Geometry check sheet. Reference: the model listing, model coordinates, mm. Round coordinates to 2 decimals unless told otherwise and drop trailing zeros. Loops run counter-clockwise (first coordinate to the right, second up) from the corner with the lowest first, then second, coordinate; pieces in that order, holes last. Notation, with made-up numbers: (75.5, 65.25) -> (85.5, 65.25) arc R25 cw to (85.5, 82.25) -> close; hole circle Ø11 at (71, 25). An arc over 180 degrees is marked (long way). Use one line per item in the form item = value.
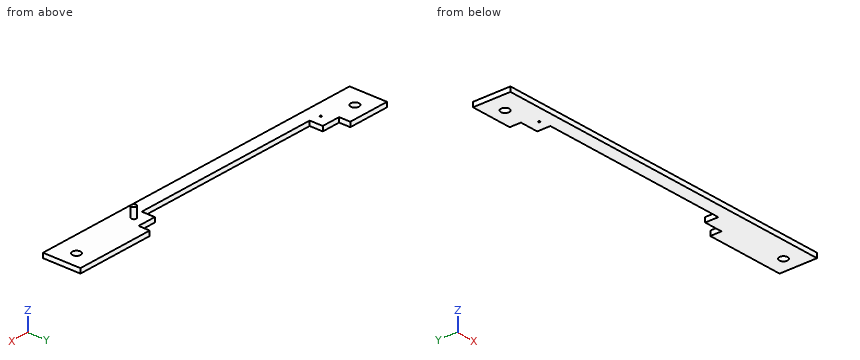
from build123d import *

# Parameters (mm, degrees)
BOX_W             = 188
BOX_H             = 20
BOX_DEPTH         = 2.5
CYLINDER_R        = 2.25
CYLINDER_DEPTH    = 2.5
CYLINDER001_R     = 2.25
CYLINDER001_DEPTH = 2.5
BOX001_W          = 123
BOX001_H          = 6
BOX001_DEPTH      = 2.5
BOX002_W          = 103
BOX002_H          = 7
BOX002_DEPTH      = 2.5
CYLINDER003_R     = 1.3
CYLINDER003_DEPTH = 6
CYLINDER004_R     = 0.5
CYLINDER004_DEPTH = 2.5


with BuildPart() as part:
    # Box → Box (join)
    with BuildSketch(Plane.XY):
        with Locations((94, 10)):
            Rectangle(BOX_W, BOX_H)
    extrude(amount=BOX_DEPTH)

    # Cylinder → Cylinder (cut)
    with BuildSketch(Plane(origin=(10.5, 12, 0), x_dir=(1, 0, 0), z_dir=(0, 0, 1))):
        Circle(CYLINDER_R)
    extrude(amount=CYLINDER_DEPTH, mode=Mode.SUBTRACT)

    # Cylinder001 → Cylinder001 (cut)
    with BuildSketch(Plane(origin=(179.5, 10.5, 0), x_dir=(1, 0, 0), z_dir=(0, 0, 1))):
        Circle(CYLINDER001_R)
    extrude(amount=CYLINDER001_DEPTH, mode=Mode.SUBTRACT)

    # Box001 → Box001 (cut)
    with BuildSketch(Plane(origin=(22.5, 14, 0), x_dir=(1, 0, 0), z_dir=(0, 0, 1))):
        with Locations((61.5, 3)):
            Rectangle(BOX001_W, BOX001_H)
    extrude(amount=BOX001_DEPTH, mode=Mode.SUBTRACT)

    # Box002 → Box002 (cut)
    with BuildSketch(Plane(origin=(32.5, 7, 0), x_dir=(1, 0, 0), z_dir=(0, 0, 1))):
        with Locations((51.5, 3.5)):
            Rectangle(BOX002_W, BOX002_H)
    extrude(amount=BOX002_DEPTH, mode=Mode.SUBTRACT)

    # Cylinder003 → Cylinder003 (join)
    with BuildSketch(Plane(origin=(141.5, 8, 2), x_dir=(1, 0, 0), z_dir=(0, 0, 1))):
        Circle(CYLINDER003_R)
    extrude(amount=CYLINDER003_DEPTH)

    # Cylinder004 → Cylinder004 (cut)
    with BuildSketch(Plane(origin=(26.75, 8, 0), x_dir=(1, 0, 0), z_dir=(0, 0, 1))):
        Circle(CYLINDER004_R)
    extrude(amount=CYLINDER004_DEPTH, mode=Mode.SUBTRACT)


solid = part.part
1. Section check B-B (z = 5.25). Record the boundary of the cut face in (x, y).
Return value:
outline = circle Ø2.6 at (141.5, 8)
2. Section check C-C (x = 91). Record the boundary of the cut face in (y, z), then the cut area to 3 significant figures.
Return value:
outline = (0, 0) -> (7, 0) -> (7, 2.5) -> (0, 2.5) -> close
area = 17.5 mm2
3. Gauge pin test, flat ends, axial feed: pin 1 (1 mm diameter, centred on y = 8.5, z = 4.5, fed in from -X); pin 2 (6 mm diameter, centred on x = 179.5, y = 10.5, fed in from +Z); pin 3 (12 mm diameter, centred on x = 26, y = 6.5, fed in from -Z); pin 4 (0.8 mm diameter, centred on x = 140, z = 1, fed in from +Y). Record the tip position at first contact, or that the pin passes through.
Return value:
pin_1 = 140.2
pin_2 = 2.5
pin_3 = 0
pin_4 = 14
4. Section check A-A (x = 10.5). Record the boundary of the cut face in (y, z), then the cut area to 4 significant figures.
Return value:
outline = (0, 0) -> (9.75, 0) -> (9.75, 2.5) -> (0, 2.5) -> close; (14.25, 0) -> (20, 0) -> (20, 2.5) -> (14.25, 2.5) -> close
area = 38.75 mm2
5. Material ranges on line 1 along Y through (x, z) = (26.75, 1.25); line 2 along Y through (x, z) = (179.5, 1.25); line 3 along Z through (x, y) = (48, 2.75), recorded low to high.
Return value:
line_1 = 0 to 7.5, 8.5 to 14
line_2 = 0 to 8.25, 12.75 to 20
line_3 = 0 to 2.5
